from build123d import *

# Parameters (mm, degrees)
BOX_W             = 20
BOX_H             = 10
BOX_DEPTH         = 10
ARRAY_COUNT       = 7
CYLINDER001_R     = 20
CYLINDER001_DEPTH = 20
CYLINDER_R        = 30
CYLINDER_DEPTH    = 100


with BuildPart() as array:
    # Box → Box (new body)
    with BuildSketch(Plane(origin=(18, -5, 90), x_dir=(1, 0, 0), z_dir=(0, 0, 1))):
        with Locations((10, 5)):
            Rectangle(BOX_W, BOX_H)
    extrude(amount=BOX_DEPTH)

    # Array: Array ×7 about axis
    array_axis = Axis((0, 0, 0), (0, 0, 1))


with BuildPart() as array_1:
    add(array.part)
    for i in range(1, ARRAY_COUNT):
        add(array.part.rotate(array_axis, i * 360 / ARRAY_COUNT))


with BuildPart() as cylinder001:
    # Cylinder001 → Cylinder001 (new body)
    with BuildSketch(Plane.XY.offset(80)):
        Circle(CYLINDER001_R)
    extrude(amount=CYLINDER001_DEPTH)


with BuildPart() as cut001:
    # Cylinder → Cylinder (new body)
    with BuildSketch(Plane.XY):
        Circle(CYLINDER_R)
    extrude(amount=CYLINDER_DEPTH)

    # Cut: cut Cylinder001
    add(cylinder001.part, mode=Mode.SUBTRACT)

    # Cut001: cut Array
    add(array_1.part, mode=Mode.SUBTRACT)


solid = cut001.part
Source: CAD feature listing. Evaluate the final solid. Frame: model axes, mm. A direction names the side the tool comes from. Round coordinates to 2 decimals unless told otherwise and drop trailing zeros. Write each loop counter-clockwise with the first axis right and the second up, starting at its lowest first coordinate (ties: lowest second). Pieces come first, ordered by that corner, then holes. Notation, with made-up numbers: (85.25, 41.5) - (102.25, 41.5) arc R27 ccw to (102.25, 74.5) - close; hole circle Ø7 at (83.5, -16.75). An arc over 180 degrees is marked (long way). Use CSV: the item, a comma, the result in double quotes. Start each with the question number.
(1) Material intervals for probe 1 along X at (y, z) = (0, 88.5); probe 2 along Y at (x, z) = (-11.5, 10); probe 3 along X at (y, z) = (0, 91.5), sorted ascending. Write a range as [from, to].
(2) Set-up query: faces 1 (the face through (25, 0, 90)), 2 (the face through (19.123, -15.96, 94.93)), 3 (the face through (0, 0, 80)), 4 (the face through (6, -25, 100)), 5 (the face through (19.123, 15.96, 94.93)). Return all of +Z, -Z, +X, -X, +Y, -Y with unobstructed straight access to the full face (end or side cutting, diameter ignored); none if empty.
(3) Cut plane D-D, the plane z = 32. Return loops of the section in (x, y), and give its area (3 significant figures).
(4) Cut plane B-B, the plane y = 0. Return loops of the section in (x, z), and give its area (3 significant figures).
(5) Cut plane C-C, the plane x = -22. Return loops of the section in (y, z).
(6) First-contact query: pin 1 Ø12 at (x, z) = (13, 84) entering from +Y; pin 2 Ø6 at (x, z) = (8, 88) entering from -Y; pin 3 Ø4 at (x, y) = (-21.5, 9) entering from +Z. Flat tips, straight axial feed; report the tip coordinate or a pass-through.
(7) Cut plane A-A, the plane z = 92.5. Return loops of the section in (x, y), and give its area (3 significant figures).
Geometry says:
1,probe 1,"[-30, -20], [20, 30]"
1,probe 2,"[-27.71, 27.71]"
1,probe 3,"[-30, -20]"
2,face 1,"+Z, +X"
2,face 2,"+Z, -Y"
2,face 3,"+Z"
2,face 4,"+Z, +X, -X, +Y, -Y"
2,face 5,"+Z, +Y"
3,outline,"circle Ø60 at (0, 0)"
3,area,"2,830 mm²"
4,outline,"(-30, 0) - (30, 0) - (30, 90) - (20, 90) - (20, 80) - (-20, 80) - (-20, 100) - (-30, 100) - close"
4,area,"5,100 mm²"
5,outline,"(-20.4, 0) - (20.4, 0) - (20.4, 100) - (16.14, 100) - (16.14, 90) - (5.05, 90) - (5.05, 100) - (-5.05, 100) - (-5.05, 90) - (-16.14, 90) - (-16.14, 100) - (-20.4, 100) - close"
6,pin 1,"y = 29.17"
6,pin 2,"y = -29.58"
6,pin 3,"z = 90"
7,outline,"(-28.82, -8.33) - (-19.62, -3.9) arc R20 cw to (-19.62, 3.9) - (-28.82, 8.33) arc R30 ccw to start; (-24.48, -17.34) arc R30 ccw to (-11.46, -27.73) - (-9.18, -17.77) arc R20 cw to (-15.28, -12.91) - close; (-24.48, 17.34) - (-15.28, 12.91) arc R20 cw to (-9.18, 17.77) - (-11.46, 27.73) arc R30 ccw to start; (-1.71, -29.95) arc R30 ccw to (14.53, -26.24) - (8.16, -18.26) arc R20 cw to (0.57, -19.99) - close; (-1.71, 29.95) - (0.57, 19.99) arc R20 cw to (8.16, 18.26) - (14.53, 26.24) arc R30 ccw to start; (15.98, -12.02) - (22.35, -20.01) arc R30 ccw to (29.58, -5) - (19.36, -5) arc R20 cw to start; (15.98, 12.02) arc R20 cw to (19.36, 5) - (29.58, 5) arc R30 ccw to (22.35, 20.01) - close"
7,area,"866 mm²"
